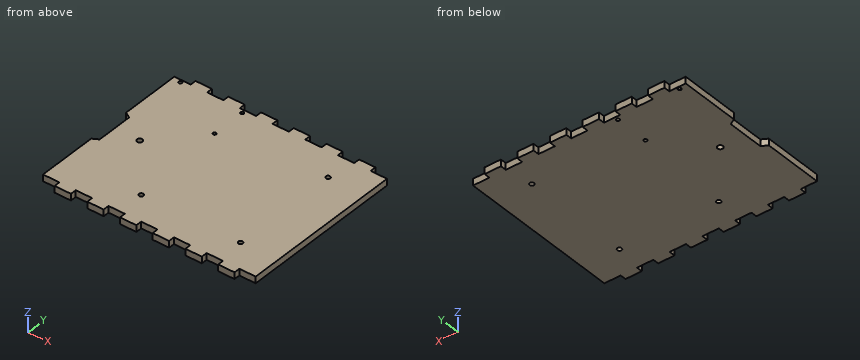
from build123d import *

# Parameters (mm, degrees)
MODEL_R             = 2.5
MODEL_R_2           = 2
MODEL_R_3           = 1.5
BOSS_EXTRUDE1_DEPTH = 6


with BuildPart() as part:
    # Model → Boss-Extrude1 (new body)
    with BuildSketch(Plane.XY):
        Polygon((206.699050252, 163.437183165), (206.699050252, 13.437183165), (191.699050252, 13.437183165), (191.699050252, 7.937183165), (176.699050252, 7.937183165), (176.699050252, 13.437183165), (161.699050252, 13.437183165), (161.699050252, 7.937183165), (146.699050252, 7.937183165), (146.699050252, 13.437183165), (131.699050252, 13.437183165), (131.699050252, 7.937183165), (116.699050252, 7.937183165), (116.699050252, 13.437183165), (101.699050252, 13.437183165), (101.699050252, 7.937183165), (86.699050252, 7.937183165), (86.699050252, 13.437183165), (71.699050252, 13.437183165), (71.699050252, 7.937183165), (56.699050252, 7.937183165), (56.699050252, 13.437183165), (41.699050252, 13.437183165), (41.699050252, 7.937183165), (26.699050252, 7.937183165), (26.699050252, 13.437183165), (11.668968128, 13.437183165), (11.668968128, 68.469250485), (17.008612601, 71.552095659), (17.008612601, 105.223573885), (11.668968128, 108.306419059), (11.668968128, 163.437183165), (26.699050252, 163.437183165), (26.699050252, 168.937183165), (41.699050252, 168.937183165), (41.699050252, 163.437183165), (56.699050252, 163.437183165), (56.699050252, 168.937183165), (71.699050252, 168.937183165), (71.699050252, 163.437183165), (86.699050252, 163.437183165), (86.699050252, 168.937183165), (101.699050252, 168.937183165), (101.699050252, 163.437183165), (116.699050252, 163.437183165), (116.699050252, 168.937183165), (131.699050252, 168.937183165), (131.699050252, 163.437183165), (146.699050252, 163.437183165), (146.699050252, 168.937183165), (161.699050252, 168.937183165), (161.699050252, 163.437183165), (176.699050252, 163.437183165), (176.699050252, 168.937183165), (191.699050252, 168.937183165), (191.699050252, 163.437183165), align=None)
        with Locations((40.168968128, 88.437183165)):
            Circle(MODEL_R, mode=Mode.SUBTRACT)
        with Locations((172.731128361, 138.437183165)):
            Circle(MODEL_R_2, mode=Mode.SUBTRACT)
        with Locations((81.699050252, 38.437183165)):
            Circle(MODEL_R_2, mode=Mode.SUBTRACT)
        with Locations((172.731128361, 38.437183165)):
            Circle(MODEL_R_2, mode=Mode.SUBTRACT)
        with Locations((76.668968128, 128.437183165)):
            Circle(MODEL_R_3, mode=Mode.SUBTRACT)
        with Locations((76.668968128, 159.937183165)):
            Circle(MODEL_R_3, mode=Mode.SUBTRACT)
        with Locations((19.18400919, 160.937183165)):
            Circle(MODEL_R_3, mode=Mode.SUBTRACT)
    extrude(amount=BOSS_EXTRUDE1_DEPTH)


solid = part.part
Design review of the part built by this model. Coordinates are the model's own, in mm. Round coordinates to 2 decimals unless told otherwise and drop trailing zeros. Loops run counter-clockwise (first coordinate to the right, second up) from the corner with the lowest first, then second, coordinate; pieces in that order, holes last. Notation, with made-up numbers: (58.5, 47) - (80.5, 47) arc R20 ccw to (80.5, 60) - close; hole circle Ø10 at (73.5, 28). An arc over 180 degrees is marked (long way). One line per item, written item: value. Start each with the question number.
1) Insertion check: pin 1 Ø3 at (y, z) = (166.5, 3.5) entering from -X; pin 2 Ø6 at (x, y) = (112, 91.5) entering from -Z; pin 3 Ø3 at (y, z) = (165.5, 4) entering from +X; pin 4 Ø1.8 at (x, z) = (168.5, 4) entering from +Y. Each pin has a flat end and moves straight along its axis. Give the tip position at first contact, or say it passes through.
2) Consider section C-C on z = 2.25. Give the number of separate pieces and of enclosed holes in the cut face, then the cut area to 3 significant figures.
3) Consider section A-A on y = 75.5. Give the boundary of the cut face in (x, z).
4) Consider section B-B on x = 111. Give the boundary of the cut face in (y, z), then the cut area to 3 significant figures.
5) To check wall thickness, follow L1, parallel to X at y = 39.5, z = 2.4; L2, parallel to Y at x = 104, z = 4.7; L3, parallel to Y at x = 78, z = 3.25. State the ranges of each line that lie inside material, in increasing order. Write a range as from..to.
Reported:
1. pin 1: stops at x = 26.7
1. pin 2: stops at z = 0
1. pin 3: stops at x = 191.7
1. pin 4: stops at y = 163.44
2. separate pieces: 1
2. enclosed holes: 7
2. area: 30,000 mm^2
3. outline: (17.01, 0) - (206.7, 0) - (206.7, 6) - (17.01, 6) - close
4. outline: (13.44, 0) - (163.44, 0) - (163.44, 6) - (13.44, 6) - close
4. area: 900 mm^2
5. L1: x = 11.67..80, 83.39..171.04, 174.43..206.7
5. L2: y = 13.44..163.44
5. L3: y = 13.44..127.75, 129.13..159.25, 160.63..163.44
